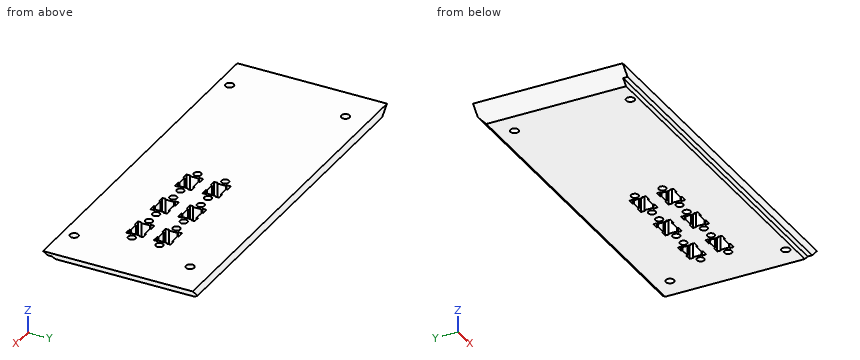
```python
from build123d import *

# Parameters (mm, degrees)
SKETCH1_W           = 200
SKETCH1_H           = 84
SKETCH1_R           = 2.25
BOSS_EXTRUDE1_DEPTH = 5
SKETCH2_W           = 200
SKETCH2_H           = 79
SKETCH2_R           = 2.25
BOSS_EXTRUDE2_DEPTH = 3
CHAMFER1_SIZE       = 8
CHAMFER3_SIZE       = 3
SKETCH3_W           = 7.071067812
SKETCH3_H           = 2.6
CUT_EXTRUDE1_DEPTH  = 234.034075139
SKETCH4_R           = 2
CUT_EXTRUDE3_DEPTH  = 218.071416819


with BuildPart() as part:
    # Sketch1 → Boss-Extrude1 (new body)
    with BuildSketch(Plane.XY):
        with Locations((100, 42)):
            Rectangle(SKETCH1_W, SKETCH1_H)
        with Locations((20, 9)):
            Circle(SKETCH1_R, mode=Mode.SUBTRACT)
        with Locations(Location((180, 9, 0), (0, 0, 180))):
            Circle(SKETCH1_R, mode=Mode.SUBTRACT)
        with Locations((20, 72)):
            Circle(SKETCH1_R, mode=Mode.SUBTRACT)
        with Locations(Location((180, 72, 0), (0, 0, 180))):
            Circle(SKETCH1_R, mode=Mode.SUBTRACT)
    extrude(amount=-BOSS_EXTRUDE1_DEPTH)

    # Sketch2 → Boss-Extrude2 (add)
    with BuildSketch(Plane(origin=(0, 0, -5), x_dir=(-1, 0, 0), z_dir=(0, 0, -1))):
        with Locations((-100, 44.5)):
            Rectangle(SKETCH2_W, SKETCH2_H)
        with Locations(Location((-20, 9, 0), (0, 0, 180))):
            Circle(SKETCH2_R, mode=Mode.SUBTRACT)
        with Locations((-180, 9)):
            Circle(SKETCH2_R, mode=Mode.SUBTRACT)
        with Locations(Location((-20, 72, 0), (0, 0, 180))):
            Circle(SKETCH2_R, mode=Mode.SUBTRACT)
        with Locations((-180, 72)):
            Circle(SKETCH2_R, mode=Mode.SUBTRACT)
    extrude(amount=BOSS_EXTRUDE2_DEPTH)

    # Chamfer1
    # the kernel refuses this chamfer: 8 mm, written as the material it takes off along each edge
    with BuildSketch(Plane(origin=(200, -15.573463904, -8), x_dir=(-0.9996219169112968, 0, -0.027495876610586296), z_dir=(0, 1, 0)), Plane(origin=(0, 104.573463904, -8), x_dir=(0.9996219169112968, 0, -0.027495876610586275), z_dir=(0, -1, 0))) as chamfer1_piece_1:
        Polygon((CHAMFER1_SIZE * 0.999621916911, CHAMFER1_SIZE * 0.0274958766106), (-CHAMFER1_SIZE * 0.0274958766106, CHAMFER1_SIZE * 0.999621916911), (0, 0), align=None)
    extrude(amount=120.146927807, mode=Mode.SUBTRACT)

    # Chamfer3
    chamfer3_edges = [part.edges().sort_by_distance(p)[0] for p in [
        (100, 84, -8),
    ]]
    chamfer(chamfer3_edges, length=CHAMFER3_SIZE)

    # Sketch3 → Cut-Extrude1 (cut, through all, along a direction that is not the sketch's normal)
    with BuildSketch(Plane(origin=(100, 0, -100), x_dir=(-0.7071067811865452, 0, -0.7071067811865498), z_dir=(0.7071067811865498, 0, -0.7071067811865452))):
        with Locations((-137.885822331, 1.3)):
            Rectangle(SKETCH3_W, SKETCH3_H)
    extrude(amount=-CUT_EXTRUDE1_DEPTH, dir=(1, 0, 0), mode=Mode.SUBTRACT)

    # Sketch4 → Cut-Extrude3 (cut, through all)
    with BuildSketch(Plane.XY):
        Polygon((165.325, 32.115271452), (165.325, 36.765271452), (166.025, 36.765271452), (166.025, 38.965271452), (162.685, 38.965271452), (162.685, 38.265271452), (157.315, 38.265271452), (157.315, 38.965271452), (153.975, 38.965271452), (153.975, 36.765271452), (154.675, 36.765271452), (154.675, 32.115271452), (153.975, 32.115271452), (153.975, 29.915271452), (157.315, 29.915271452), (157.315, 30.615271452), (162.685, 30.615271452), (162.685, 29.915271452), (166.025, 29.915271452), (166.025, 32.115271452), align=None)
        Polygon((140.325, 32.115271452), (140.325, 36.765271452), (141.025, 36.765271452), (141.025, 38.965271452), (137.685, 38.965271452), (137.685, 38.265271452), (132.315, 38.265271452), (132.315, 38.965271452), (128.975, 38.965271452), (128.975, 36.765271452), (129.675, 36.765271452), (129.675, 32.115271452), (128.975, 32.115271452), (128.975, 29.915271452), (132.315, 29.915271452), (132.315, 30.615271452), (137.685, 30.615271452), (137.685, 29.915271452), (141.025, 29.915271452), (141.025, 32.115271452), align=None)
        Polygon((115.325, 32.115271452), (115.325, 36.765271452), (116.025, 36.765271452), (116.025, 38.965271452), (112.685, 38.965271452), (112.685, 38.265271452), (107.315, 38.265271452), (107.315, 38.965271452), (103.975, 38.965271452), (103.975, 36.765271452), (104.675, 36.765271452), (104.675, 32.115271452), (103.975, 32.115271452), (103.975, 29.915271452), (107.315, 29.915271452), (107.315, 30.615271452), (112.685, 30.615271452), (112.685, 29.915271452), (116.025, 29.915271452), (116.025, 32.115271452), align=None)
        Polygon((140.325, 47.115271452), (140.325, 51.765271452), (141.025, 51.765271452), (141.025, 53.965271452), (137.685, 53.965271452), (137.685, 53.265271452), (132.315, 53.265271452), (132.315, 53.965271452), (128.975, 53.965271452), (128.975, 51.765271452), (129.675, 51.765271452), (129.675, 47.115271452), (128.975, 47.115271452), (128.975, 44.915271452), (132.315, 44.915271452), (132.315, 45.615271452), (137.685, 45.615271452), (137.685, 44.915271452), (141.025, 44.915271452), (141.025, 47.115271452), align=None)
        Polygon((115.325, 47.115271452), (115.325, 51.765271452), (116.025, 51.765271452), (116.025, 53.965271452), (112.685, 53.965271452), (112.685, 53.265271452), (107.315, 53.265271452), (107.315, 53.965271452), (103.975, 53.965271452), (103.975, 51.765271452), (104.675, 51.765271452), (104.675, 47.115271452), (103.975, 47.115271452), (103.975, 44.915271452), (107.315, 44.915271452), (107.315, 45.615271452), (112.685, 45.615271452), (112.685, 44.915271452), (116.025, 44.915271452), (116.025, 47.115271452), align=None)
        Polygon((165.325, 47.115271452), (165.325, 51.765271452), (166.025, 51.765271452), (166.025, 53.965271452), (162.685, 53.965271452), (162.685, 53.265271452), (157.315, 53.265271452), (157.315, 53.965271452), (153.975, 53.965271452), (153.975, 51.765271452), (154.675, 51.765271452), (154.675, 47.115271452), (153.975, 47.115271452), (153.975, 44.915271452), (157.315, 44.915271452), (157.315, 45.615271452), (162.685, 45.615271452), (162.685, 44.915271452), (166.025, 44.915271452), (166.025, 47.115271452), align=None)
        with Locations((151.175, 34.440271452)):
            Circle(SKETCH4_R)
        with Locations(Location((168.825, 34.440271452, 0), (0, 0, 180))):
            Circle(SKETCH4_R)
        with Locations((126.175, 34.440271452)):
            Circle(SKETCH4_R)
        with Locations(Location((143.825, 34.440271452, 0), (0, 0, 180))):
            Circle(SKETCH4_R)
        with Locations((101.175, 34.440271452)):
            Circle(SKETCH4_R)
        with Locations(Location((118.825, 34.440271452, 0), (0, 0, 180))):
            Circle(SKETCH4_R)
        with Locations((126.175, 49.440271452)):
            Circle(SKETCH4_R)
        with Locations((143.825, 49.440271452)):
            Circle(SKETCH4_R)
        with Locations((101.175, 49.440271452)):
            Circle(SKETCH4_R)
        with Locations(Location((118.825, 49.440271452, 0), (0, 0, 180))):
            Circle(SKETCH4_R)
        with Locations((151.175, 49.440271452)):
            Circle(SKETCH4_R)
        with Locations(Location((168.825, 49.440271452, 0), (0, 0, 180))):
            Circle(SKETCH4_R)
    extrude(amount=-CUT_EXTRUDE3_DEPTH, mode=Mode.SUBTRACT)


solid = part.part
```
The listing builds one solid part. Answer for the finished solid, in the listing's coordinates (mm). Coordinates: 2 decimals unless noted, no trailing zeros. Write each loop counter-clockwise with the first axis right and the second up, starting at its lowest first coordinate (ties: lowest second). Pieces come first, ordered by that corner, then holes. Notation, with made-up numbers: (-35.75, -15.75) - (10.25, -15.75) arc R29 ccw to (10.25, 22.25) - close; hole circle Ø6 at (-3.75, 64.25). An arc over 180 degrees is marked (long way). Return JSON: item names as keys, results as strings. Group by question number.
1. A cutting plane is placed at D-D, the plane z = -2. Give the number of separate pieces and of enclosed holes in the cut face, plus the area to 3 significant figures.
2. A cutting plane is placed at B-B, the plane x = 20. Determine the outline of the cut face in (y, z).
3. A cutting plane is placed at C-C, the plane y = 26. Determine the outline of the cut face in (x, z), plus the area to 3 significant figures.
4. Straight lines are drawn through the part: L1, parallel to Y at x = 162.5, z = -0.25; L2, parallel to Y at x = 138, z = -4.75; L3, parallel to X at y = 8, z = -2. For each, find the intervals that lie inside material, in ascending order.
5. A cutting plane is placed at A-A, the plane y = 72. Determine the outline of the cut face in (x, z).
6. Given pin 1 (1.5 mm diameter, centred on y = 20.5, z = -5.5, fed in from +X); pin 2 (0.7 mm diameter, centred on y = 31.5, z = -3.5, fed in from -X); pin 3 (0.6 mm diameter, centred on y = 38.5, z = -5.5, fed in from +X), each flat-ended and moving along its own axis, determine where each tip first touches the part or whether it passes through.
Ans:
{
 "1": {"separate pieces": "1", "enclosed holes": "22", "area": "15,200 mm²"},
 "2": {"outline": "(2.6, -5) - (5, -5) - (5, -8) - (6.75, -8) - (6.75, 0) - (2.6, 0) - close; (11.25, -8) - (69.75, -8) - (69.75, 0) - (11.25, 0) - close; (74.25, -8) - (81, -8) - (84, -5) - (84, 0) - (74.25, 0) - close"},
 "3": {"outline": "(0, 0) - (8, -8) - (192, -8) - (200, 0) - close", "area": "1,540 mm²"},
 "4": {"L1": "2.6 to 30.62, 38.27 to 45.62, 53.27 to 84", "L2": "2.6 to 29.92, 38.97 to 44.92, 53.97 to 84", "L3": "2 to 17.98, 22.02 to 177.98, 182.02 to 198"},
 "5": {"outline": "(0, 0) - (8, -8) - (17.75, -8) - (17.75, 0) - close; (22.25, -8) - (177.75, -8) - (177.75, 0) - (22.25, 0) - close; (182.25, -8) - (192, -8) - (200, 0) - (182.25, 0) - close"},
 "6": {"pin 1": "x = 195.25", "pin 2": "x = 3.15", "pin 3": "x = 194.8"}
}
